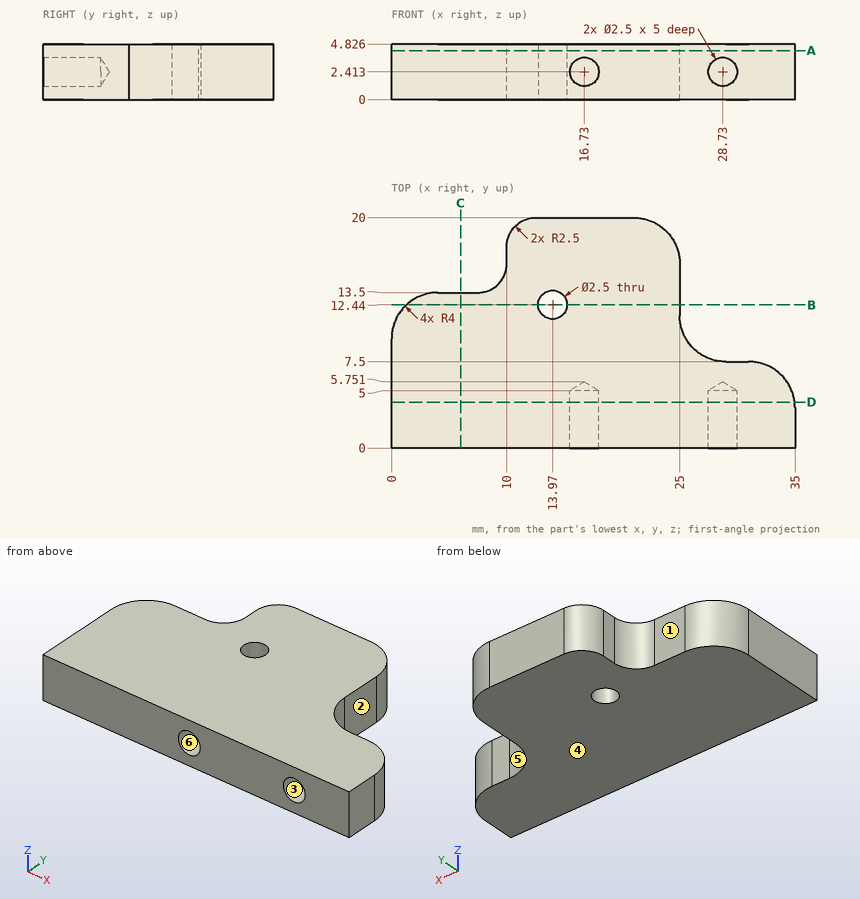
Part print with two shaded views. Sizes in mm from the minimum x, y, z corner. A direction names the side the tool comes from. Coordinates: 2 decimals unless noted, no trailing zeros. Order: outer loops, then holes, each group sorted by start corner. A loop starts at its lowest first (then second) coordinate and runs counter-clockwise, first axis right, second up. Notation, with made-up numbers: M -5.75,-27 L 47.25,-27 A23 cw 47.25,9 Z; hole C 80,83.5 d1. An arc over 180 degrees is marked long. One line per question, with ' | ' between items. Start each with the question number.
1. Wall check: line 1 along Z through (x, y) = (28.73, 1.4); line 2 along Y through (x, z) = (13.5, 3.45); line 3 along Y through (x, z) = (24, 4.35) (1 decimal). Give the ranges that are in metal, low to high. Write a range as [from, to].
2. Mould opens along Z. For the marked faces 4, 5 and 6 say: +Z half, -Z half, draft (parallel to the pull), parting line (faces both ways), or undercut.
3. Cut at C-C (x = 6). Write the cut outline in (y, z).
4. Cut at A-A (z = 4.25). Write the cut outline in (x, y), plus the area to 3 significant figures.
5. Flat gauge pins, fed straight in: P1, Ø1, axis at x = 29.5, z = 2, coming from the +Y side; P2, Ø1.6, axis at y = 16.5, z = 1.5, coming from the -X side; P3, Ø2, axis at x = 13.97, y = 12.44, coming from the -Z side; P4, Ø1.5, axis at x = 28.73, z = 2.413, coming from the -Y side. Where does each tip first touch, or does it go through?
6. Cut at B-B (y = 12.44). Write the cut outline in (x, z).
7. Tool access for the marked faces 1, 2 and 3: list every direction of +Z, -Z, +X, -X, +Y, -Y with a clear straight run to the whole face (end or side of a thin tool).
8. Cut at D-D (y = 4). Write the cut outline in (x, z).
The answers:
1) line 1: z = [0, 1.16], [3.66, 4.83] | line 2: y = [0, 11.28], [13.6, 20] | line 3: y = [0, 18.6]
2) face 4: -Z half | face 5: draft | face 6: undercut
3) outline: M 0,0 L 13.5,0 L 13.5,4.83 L 0,4.83 Z
4) outline: M 0,0 L 35,0 L 35,3.5 A4 ccw 31,7.5 L 29,7.5 A4 cw 25,11.5 L 25,16 A4 ccw 21,20 L 12.5,20 A2.5 ccw 10,17.5 L 10,16 A2.5 cw 7.5,13.5 L 4,13.5 A4 ccw 0,9.5 Z; hole C 13.97,12.44 d2.5 | area: 498 mm2
5) P1: stops at y = 7.5 | P2: stops at x = 9.98 | P3: passes through | P4: stops at y = 5.3
6) outline: M 1.29,0 L 12.72,0 L 12.72,4.83 L 1.29,4.83 Z; M 15.22,0 L 25,0 L 25,4.83 L 15.22,4.83 Z
7) face 1: +Z, -Z, -X, +Y | face 2: +Z, -Z, +X, +Y | face 3: -Y
8) outline: M 0,0 L 34.97,0 L 34.97,4.83 L 0,4.83 Z; hole C 16.73,2.41 d2.5; hole C 28.73,2.41 d2.5
